Input: part model. Units: mm. Frame: model coordinates. A direction names the side the tool comes from. Give positions to 0.01 mm unless a question says otherwise; leave off trailing zeros. Order: outer loops, then holes, each group sorted by start corner. A loop starts at its lowest first (then second) coordinate and runs counter-clockwise, first axis right, second up. Notation, with made-up numbers: (62.25, 83.5) - (98.25, 83.5) arc R36 ccw to (98.25, 122.5) - close; hole circle Ø3 at (31, 79). An arc over 180 degrees is marked (long way). Answer in a Markdown table with one row per item. Add a question column.
1. Access query for faces 4 (the face through (5.4, 35.1, -15.9)), 5 (the face through (10.496, 3.8, 31)), 6 (the face through (20.016, 4.93, 23.79)). Directions: +Z, -Z, +X, -X, +Y, -Y. A direction counts if a zero-diameter tool reaches every point of the face in a straight line with its end or side. Return the directions, or none.
2. Section query D-D on x = 37.5. Return loops of the section in (y, z).
3. Contact query for flat-ended pins moving along their axis: pin 1 (3 mm diameter, centred on x = 8, y = 6, fed in from +Z); pin 2 (2 mm diameter, centred on y = 5, z = 31.77, fed in from -X); pin 3 (19 mm diameter, centred on x = 74, z = 60, fed in from +Y); pin 4 (3 mm diameter, centred on x = 19.5, y = 6.5, fed in from +Z). Output: stop coordinate, or through.
4. Section query C-C on z = 0. Return loops of the section in (x, y).
5. Ray query, line 1 (Z direction, x = 13.5, y = 4); line 2 (Y direction, x = 27.5, z = -17); line 3 (X direction, y = 8, z = 0). Return the intervals inside material, ascending. Write a range as [from, to].
6. Section query A-A on x = 76.5. Return loops of the section in (y, z), and give its area (3 significant figures).
7. Section query B-B on y = 5. Return loops of the section in (x, z), and give its area (3 significant figures).
8. Mould query, pull axis X, two halves, no side actions, for faces 1 (the face through (84.49, 4.93, 70.72)), 2 (the face through (74.46, 4.93, 49.46)), 3 (the face through (61.273, 4.93, 70.489)). Classes: released by +X, released by -X, zero draft, split by the parting line, or undercut.
```python
from build123d import *

# Parameters (mm, degrees)
SKETCH1_R           = 7.55
SKETCH1_R_2         = 5
SKETCH1_R_3         = 10.55
BOSS_EXTRUDE1_DEPTH = 10
SKETCH2_R           = 1.25
CUT_EXTRUDE1_DEPTH  = 10
SKETCH4_R           = 7.5
BOSS_EXTRUDE2_DEPTH = 30
BOSS_EXTRUDE2_TAPER = 7
SKETCH5_R           = 1.25
CUT_EXTRUDE2_DEPTH  = 10
FILLET1_R           = 15
FILLET2_R           = 7.5


with BuildPart() as part:
    # Sketch1 → Boss-Extrude1 (new body)
    with BuildSketch(Plane(origin=(0, 0, 0), x_dir=(1, 0, 0), z_dir=(0, 1, 0))):
        Polygon((23.995878661, -35), (56.995878661, -35), (56.995878661, -75), (88.995878661, -75), (88.995878661, -25), (88.995878661, 25), (17.5, 25), (-2.004121339, 25), (-2.004121339, 7.840472806), (23.995878661, 7.840472806), (23.995878661, 0), (23.995878661, -28.53803828), (10.495878661, -28.53803828), (10.495878661, -35), align=None)
        with Locations(Location((73.995878661, 0, 0), (0, 0, 270))):
            Circle(SKETCH1_R, mode=Mode.SUBTRACT)
        with Locations(Location((51.495878661, 0, 0), (0, 0, 270))):
            Circle(SKETCH1_R_2, mode=Mode.SUBTRACT)
        with Locations(Location((73.995878661, -60, 0), (0, 0, 270))):
            Circle(SKETCH1_R_3, mode=Mode.SUBTRACT)
    extrude(amount=BOSS_EXTRUDE1_DEPTH)

    # Sketch2 → Cut-Extrude1 (cut)
    with BuildSketch(Plane.ZY.offset(-10.495878661)):
        with Locations((31.76901914, 5)):
            Circle(SKETCH2_R)
    extrude(amount=-CUT_EXTRUDE1_DEPTH, mode=Mode.SUBTRACT)

    # Sketch4 → Boss-Extrude2 (add)
    with BuildSketch(Plane(origin=(0, 10, 0), x_dir=(1, 0, 0), z_dir=(0, 1, 0))):
        with Locations((6.495878661, 16.5)):
            Circle(SKETCH4_R)
    extrude(amount=BOSS_EXTRUDE2_DEPTH, taper=BOSS_EXTRUDE2_TAPER)

    # Sketch5 → Cut-Extrude2 (cut)
    with BuildSketch(Plane(origin=(0, 40, 0), x_dir=(1, 0, 0), z_dir=(0, 1, 0))):
        with Locations(Location((6.495878661, 16.5, 0), (0, 0, 270))):
            Circle(SKETCH5_R)
    extrude(amount=-CUT_EXTRUDE2_DEPTH, mode=Mode.SUBTRACT)

    # Fillet1
    # the kernel refuses this fillet: 15 mm, written as the material it adds along each edge
    with BuildSketch(Plane(origin=(56.995878661, 0, 35), x_dir=(-1, 0, 0), z_dir=(0, 1, 0)), Plane(origin=(23.995878661, 0, -7.840472806), x_dir=(-1, 0, 0), z_dir=(0, 1, 0))) as fillet1_piece_1:
        with BuildLine():
            CenterArc((FILLET1_R, FILLET1_R), FILLET1_R, 180, 90)
            Line((0, FILLET1_R), (0, 0))
            Line((0, 0), (FILLET1_R, 0))
        make_face()
    extrude(amount=10)
    with BuildSketch(Plane(origin=(23.995878661, 0, 28.53803828), x_dir=(0, 0, -1), z_dir=(0, 1, 0))) as fillet1_piece_2:
        with BuildLine():
            CenterArc((14.924811557, 15), FILLET1_R, 185.739170477, 84.260829523)
            Line((0, 13.5), (0, 0))
            Line((0, 0), (14.924811557, 0))
        make_face()
    extrude(amount=10)
    # the kernel refuses this fillet: 15 mm, written as the material it takes off along each edge
    with BuildSketch(Plane(origin=(88.995878661, -37.5, -25), x_dir=(0, 0, 1), z_dir=(0, 1, 0)), Plane(origin=(88.995878661, -37.5, 75), x_dir=(-1, 0, 0), z_dir=(0, 1, 0)), Plane(origin=(56.995878661, -37.5, 75), x_dir=(0, 0, -1), z_dir=(0, 1, 0))) as fillet1_2_piece_1:
        with BuildLine():
            CenterArc((FILLET1_R, -FILLET1_R), FILLET1_R, 90, 90)
            Line((0, -FILLET1_R), (0, 0))
            Line((0, 0), (FILLET1_R, 0))
        make_face()
    extrude(amount=85, mode=Mode.SUBTRACT)

    # Fillet2
    fillet2_edges = [part.edges().sort_by_distance(p)[0] for p in [
        (-2.004121339, 5, -7.840472806),
        (-2.004121339, 5, -25),
    ]]
    fillet(fillet2_edges, radius=FILLET2_R)


solid = part.part
```
Answer:
| question | item | result |
|---|---|---|
| 1 | face 4 | +Y |
| 1 | face 5 | +Z, -X, +Y, -Y |
| 1 | face 6 | -X, +Y, -Y |
| 2 | outline | (0, -25) - (10, -25) - (10, 35) - (0, 35) - close |
| 3 | pin 1 | stops at z = -7.83 |
| 3 | pin 2 | stops at x = 20.5 |
| 3 | pin 3 | passes through |
| 3 | pin 4 | stops at z = 35 |
| 4 | outline | (22.18, 0) - (46.5, 0) - (46.5, 10) - (22.18, 10) - close; (56.5, 0) - (66.45, 0) - (66.45, 10) - (56.5, 10) - close; (81.55, 0) - (89, 0) - (89, 10) - (81.55, 10) - close |
| 5 | line 1 | z = [-25, -7.15], [27.92, 31.02], [32.52, 35] |
| 5 | line 2 | y = [0, 10] |
| 5 | line 3 | x = [22.18, 46.5], [56.5, 66.45], [81.55, 89] |
| 6 | outline | (0, -24.79) - (10, -24.79) - (10, -7.12) - (0, -7.12) - close; (0, 7.12) - (10, 7.12) - (10, 49.75) - (0, 49.75) - close; (0, 70.25) - (10, 70.25) - (10, 74.79) - (0, 74.79) - close |
| 6 | area | 648 mm² |
| 7 | outline | (-2, -17.5) arc R7.5 ccw to (5.5, -25) - (74, -25) arc R15 ccw to (89, -10) - (89, 60) arc R15 ccw to (74, 75) - (72, 75) arc R15 ccw to (57, 60) - (57, 50) arc R15 cw to (42, 35) - (10.5, 35) - (10.5, 33.02) - (20.5, 33.02) - (20.5, 30.52) - (10.5, 30.52) - (10.5, 28.54) arc R15 cw to (24, 13.61) - (24, 7.16) arc R15 cw to (9, -7.84) - (5.5, -7.84) arc R7.5 ccw to (-2, -15.34) - close; hole circle Ø10 at (51.5, 0); hole circle Ø21.1 at (74, 60); hole circle Ø15.1 at (74, 0) |
| 7 | area | 5,060 mm² |
| 8 | face 1 | released by +X |
| 8 | face 2 | undercut |
| 8 | face 3 | released by -X |
